Part model, mm, in its own coordinate system. Coordinates: 2 decimals unless noted, no trailing zeros. Loops run counter-clockwise (first coordinate to the right, second up) from the corner with the lowest first, then second, coordinate; pieces in that order, holes last. Notation, with made-up numbers: M 59,4 L 77,4 A20 cw 77,28 Z; hole C -18.5,-17 d2. An arc over 180 degrees is marked long. Use CSV: the item, a comma, the result in double quotes. Start each with the question number.
from build123d import *

# Parameters (mm, degrees)
BOSS_EXTRU_1_DEPTH         = 1
ESQUISSE2_R                = 1.5
ENL_V_MAT_EXTRU_1_DEPTH    = 2
R_P_TITION_LIN_AIRE1_COUNT = 3
R_P_TITION_LIN_AIRE1_PITCH = 10
R_P_TITION_LIN_AIRE2_COUNT = 3
R_P_TITION_LIN_AIRE2_PITCH = 10
R_P_TITION_LIN_AIRE3_COUNT = 4
R_P_TITION_LIN_AIRE3_PITCH = 10


with BuildPart() as part:
    # Esquisse1 → Boss.-Extru.1 (new body)
    with BuildSketch(Plane.XY):
        Polygon((-25, 10), (25, 10), (25, 0), (5, 0), (5, -30), (-5, -30), (-5, 0), (-25, 0), align=None)
    extrude(amount=BOSS_EXTRU_1_DEPTH)

    # Esquisse2 → Enlèv. mat.-Extru.1 (cut, through all)
    with BuildSketch(Plane.XY.offset(1)):
        with Locations((0, 5)):
            Circle(ESQUISSE2_R)
    enl_v_mat_extru_1 = extrude(amount=-ENL_V_MAT_EXTRU_1_DEPTH, mode=Mode.SUBTRACT)

    # Répétition linéaire1: Enlèv. mat.-Extru.1 ×3
    with Locations(*[(-i * R_P_TITION_LIN_AIRE1_PITCH, 0, 0) for i in range(1, R_P_TITION_LIN_AIRE1_COUNT)]):
        add(enl_v_mat_extru_1, mode=Mode.SUBTRACT)

    # Répétition linéaire2: Enlèv. mat.-Extru.1 ×3
    with Locations(*[(i * R_P_TITION_LIN_AIRE2_PITCH, 0, 0) for i in range(1, R_P_TITION_LIN_AIRE2_COUNT)]):
        add(enl_v_mat_extru_1, mode=Mode.SUBTRACT)

    # Répétition linéaire3: Enlèv. mat.-Extru.1 ×4
    with Locations(*[(0, -i * R_P_TITION_LIN_AIRE3_PITCH, 0) for i in range(1, R_P_TITION_LIN_AIRE3_COUNT)]):
        add(enl_v_mat_extru_1, mode=Mode.SUBTRACT)


solid = part.part
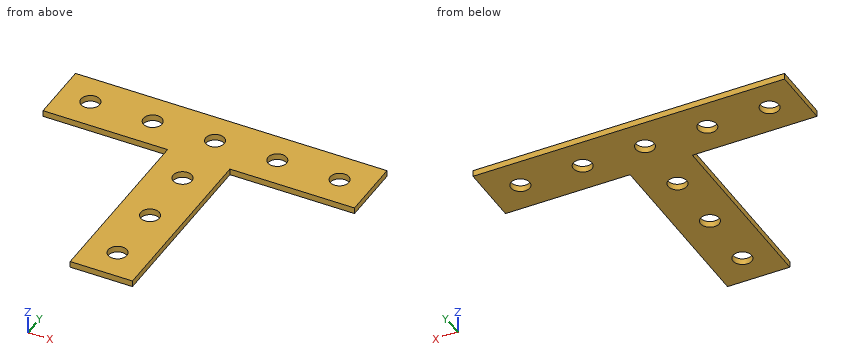
1. Slice it at C-C, the plane y = 5. List the corners of the cut face in (x, z).
2. Pin check, flat tips, straight feed: pin 1 (8 mm diameter, centred on x = 10, y = -23, fed in from +Z); pin 2 (4 mm diameter, centred on x = -20, y = 5, fed in from -Z). Stop position of each tip, or through.
3. Wall check: probe 1 along Y at (x, z) = (0, 0.3); probe 2 along Y at (x, z) = (-10, 0.25); probe 3 along Y at (x, z) = (14.5, 0.6). Give the ranges that are in metal, low to high.
4. Slice it at A-A, the plane y = -25. List the corners of the cut face in (x, z), and give its area (3 significant figures).
5. Slice it at D-D, the plane z = 0.8. State how many separate pieces and enclosed holes the cut face has, and give its area (3 significant figures).
6. Slice it at B-B, the plane x = 0. List the corners of the cut face in (y, z), and give its area (3 significant figures).
Found:
1,outline,"M -25,0 L -21.5,0 L -21.5,1 L -25,1 Z; M -18.5,0 L -11.5,0 L -11.5,1 L -18.5,1 Z; M -8.5,0 L -1.5,0 L -1.5,1 L -8.5,1 Z; M 1.5,0 L 8.5,0 L 8.5,1 L 1.5,1 Z; M 11.5,0 L 18.5,0 L 18.5,1 L 11.5,1 Z; M 21.5,0 L 25,0 L 25,1 L 21.5,1 Z"
2,pin 1,"through"
2,pin 2,"z = 0"
3,probe 1,"-30 to -26.5, -23.5 to -16.5, -13.5 to -6.5, -3.5 to 3.5, 6.5 to 10"
3,probe 2,"0 to 3.5, 6.5 to 10"
3,probe 3,"0 to 10"
4,outline,"M -5,0 L -1.5,0 L -1.5,1 L -5,1 Z; M 1.5,0 L 5,0 L 5,1 L 1.5,1 Z"
4,area,"7.00 mm^2"
5,separate pieces,"1"
5,enclosed holes,"8"
5,area,"743 mm^2"
6,outline,"M -30,0 L -26.5,0 L -26.5,1 L -30,1 Z; M -23.5,0 L -16.5,0 L -16.5,1 L -23.5,1 Z; M -13.5,0 L -6.5,0 L -6.5,1 L -13.5,1 Z; M -3.5,0 L 3.5,0 L 3.5,1 L -3.5,1 Z; M 6.5,0 L 10,0 L 10,1 L 6.5,1 Z"
6,area,"28.0 mm^2"
